The listing builds one solid part. Answer for the finished solid, in the listing's coordinates (mm). Face numbers are marked on the shaded views. A direction names the side the tool comes from. Coordinates: 2 decimals unless noted, no trailing zeros. Loops run counter-clockwise (first coordinate to the right, second up) from the corner with the lowest first, then second, coordinate; pieces in that order, holes last. Notation, with made-up numbers: (-18, 8) - (23, 8) arc R22 cw to (23, 28) - close; hole circle Ø4 at (5.5, -29). An arc over 180 degrees is marked (long way). Write each question's results on one line, items separated by ' | '. Start each with the question number.
(1) Find section C-C on x = -5. Determine the outline of the cut face in (y, z).
(2) Find section B-B on z = -2.25. Determine the outline of the cut face in (x, y), then the cut area to 3 significant figures.
(3) Determine the mould class of the marked faces 3, 4 and 5 for opening direction X: released by +X, released by -X, zero draft, split by the parting line, or undercut.
(4) For the marked faces 1 and 2, determine the directions among +Z, -Z, +X, -X, +Y, -Y from which every point of the face is accessible in a straight line to the end or side of a thin tool.
(5) Given pin 1 Ø1.9 at (x, y) = (8.5, -5) entering from +Z; pin 2 Ø3 at (x, y) = (18, 1.5) entering from +Z; pin 3 Ø3 at (x, y) = (-16.5, 0) entering from +Z, each flat-ended and moving along its own axis, determine where each tip first touches the part or whether it passes through.
(6) Find section A-A on y = 2.5. Determine the outline of the cut face in (x, z), then the cut area to 4 significant figures.
(7) Find section D-D on y = -4.5. Determine the outline of the cut face in (x, z).
(8) Consider line 1 (X direction, y = 4, z = 6); line 2 (Y direction, x = -11, z = 5.5); line 3 (X direction, y = -1, z = 5). Determine where each line is inside the solid, lowest interval first. Write a range as from..to.
from build123d import *

# Parameters (mm, degrees)
F0_W     = 46.5
F0_H     = 26.5
F0_W_2   = 38.5
F0_H_2   = 18.5
F1_DEPTH = 8
F2_W     = 46.5
F2_H     = 26.5
F3_DEPTH = 4
F4_W     = 40
F4_H     = 9.5
F5_DEPTH = 3
F6_W     = 23
F6_H     = 6
F7_DEPTH = 2.5
F8_R     = 3


with BuildPart() as f1:
    # F0 (on Top) → F1 (new body)
    with BuildSketch(Plane.XY):
        Rectangle(F0_W, F0_H)
        Rectangle(F0_W_2, F0_H_2, mode=Mode.SUBTRACT)
    extrude(amount=F1_DEPTH)

    # F2 (on face) → F3 (join)
    with BuildSketch(Plane(origin=(0, 0, 0), x_dir=(1, 0, 0), z_dir=(0, 0, -1))):
        Rectangle(F2_W, F2_H)
    extrude(amount=F3_DEPTH)

    # F4 (on Front) → F5 (cut, symmetric)
    with BuildSketch(Plane.XZ):
        with Locations((-0.75, 3.25)):
            Rectangle(F4_W, F4_H)
    extrude(amount=F5_DEPTH, both=True, mode=Mode.SUBTRACT)

    # F6 (on face) → F7 (cut, through all)
    with BuildSketch(Plane.XY.offset(-1.5)):
        with Locations((3.75, 0)):
            Rectangle(F6_W, F6_H)
    extrude(amount=-F7_DEPTH, mode=Mode.SUBTRACT)

    # F8
    f8_edges = [f1.edges().sort_by_distance(p)[0] for p in [
        (-23.25, -13.25, 2),
        (23.25, -13.25, 2),
        (-23.25, 13.25, 2),
        (23.25, 13.25, 2),
    ]]
    fillet(f8_edges, radius=F8_R)


solid = f1.part
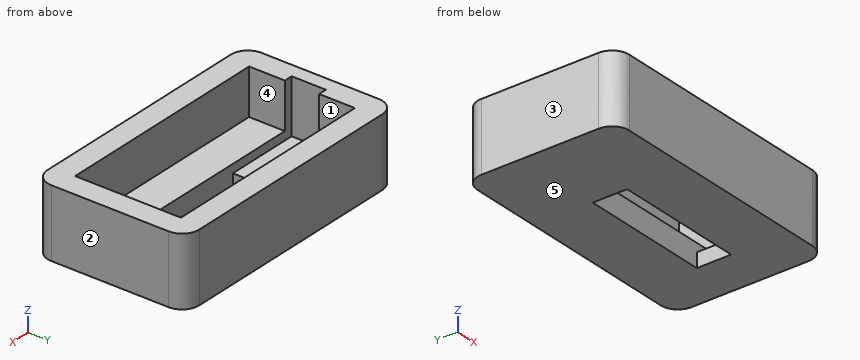
Values:
1) outline: (-13.25, -4) - (-3, -4) - (-3, 0) - (-9.25, 0) - (-9.25, 8) - (-13.25, 8) - close; (3, -4) - (13.25, -4) - (13.25, 8) - (9.25, 8) - (9.25, 0) - (3, 0) - close
2) outline: (-23.25, -10.25) arc R3 ccw to (-20.25, -13.25) - (20.25, -13.25) arc R3 ccw to (23.25, -10.25) - (23.25, 10.25) arc R3 ccw to (20.25, 13.25) - (-20.25, 13.25) arc R3 ccw to (-23.25, 10.25) - close; hole (-7.75, -3) - (15.25, -3) - (15.25, 3) - (-7.75, 3) - close | area: 1,090 mm²
3) face 3: released by -X | face 4: undercut | face 5: zero draft
4) face 1: +Z | face 2: +Z, -Z, +X, +Y, -Y
5) pin 1: stops at z = 0 | pin 2: stops at z = 8 | pin 3: stops at z = -1.5
6) outline: (-23.25, -4) - (-7.75, -4) - (-7.75, -1.5) - (-20.75, -1.5) - (-20.75, 8) - (-23.25, 8) - close; (15.25, -4) - (23.25, -4) - (23.25, 8) - (19.25, 8) - (19.25, -1.5) - (15.25, -1.5) - close | area: 120.5 mm²
7) outline: (-23.25, -4) - (23.25, -4) - (23.25, 8) - (19.25, 8) - (19.25, 0) - (-19.25, 0) - (-19.25, 8) - (-23.25, 8) - close
8) line 1: x = -23.25..-19.25, 19.25..23.25 | line 2: y = -13.25..-9.25, 9.25..13.25 | line 3: x = -23.25..-20.75, 19.25..23.25
